Verification items for this drawing (mm, ordinates from the low corner). Round coordinates to 2 decimals unless told otherwise and drop trailing zeros. Order: outer loops, then holes, each group sorted by start corner. A loop starts at its lowest first (then second) coordinate and runs counter-clockwise, first axis right, second up. Notation, with made-up numbers: (65.25, 28.5) -> (87.25, 28.5) arc R20 ccw to (87.25, 45.5) -> close; hole circle Ø4 at (69, 89.25). An arc over 180 degrees is marked (long way). Put each result on its own line as item: value.
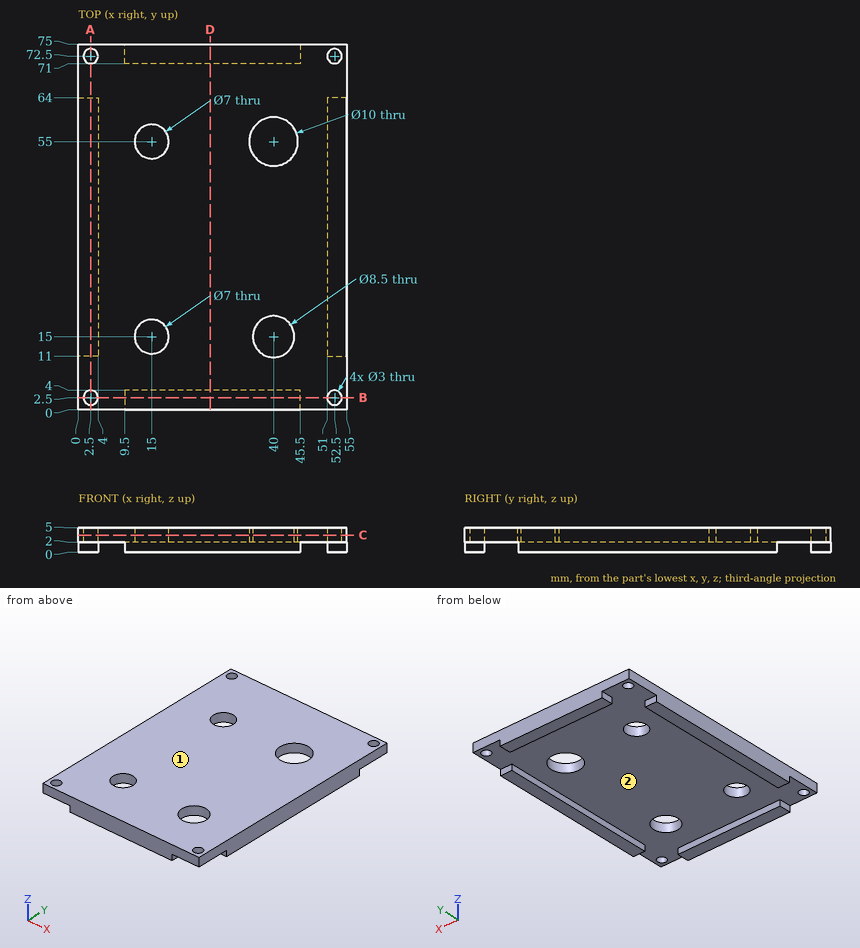
Item 1: Section check C-C on z = 3.5. State how many separate pieces and enclosed holes the cut face has, then the cut area to 3 significant figures.
Check sheet entries:
separate pieces: 1
enclosed holes: 8
area: 3,880 mm^2
Item 2: Section check D-D on x = 27. Record the boundary of the cut face in (y, z).
Check sheet entries:
outline: (0, 0) -> (4, 0) -> (4, 2) -> (71, 2) -> (71, 0) -> (75, 0) -> (75, 5) -> (0, 5) -> close
Item 3: Section check B-B on y = 2.5. Record the boundary of the cut face in (x, z).
Check sheet entries:
outline: (0, 2) -> (1, 2) -> (1, 5) -> (0, 5) -> close; (4, 2) -> (9.5, 2) -> (9.5, 0) -> (45.5, 0) -> (45.5, 2) -> (51, 2) -> (51, 5) -> (4, 5) -> close; (54, 2) -> (55, 2) -> (55, 5) -> (54, 5) -> close
Item 4: Material ranges on L1, parallel to Y at x = 2.5, z = 3.8; L2, parallel to Y at x = 40, z = 2.85; L3, parallel to X at y = 72.5, z = 4.15, recorded low to high. Write a range as [from, to].
Check sheet entries:
L1: y = [0, 1], [4, 71], [74, 75]
L2: y = [0, 10.75], [19.25, 50], [60, 75]
L3: x = [0, 1], [4, 51], [54, 55]
Item 5: Gauge pin test, flat ends, axial feed: pin 1 Ø1.6 at (y, z) = (72.5, 1) entering from +X; pin 2 Ø2 at (x, y) = (16, 34.5) entering from -Z; pin 3 Ø1 at (x, z) = (1.5, 0.5) entering from +Y; pin 4 Ø2.5 at (x, y) = (52.5, 72.5) entering from -Z. Record the tip position at first contact, or that the pin passes through.
Check sheet entries:
pin 1: stops at x = 45.5
pin 2: stops at z = 2
pin 3: stops at y = 64
pin 4: passes through
Item 6: Section check A-A on x = 2.5. Record the boundary of the cut face in (y, z).
Check sheet entries:
outline: (0, 2) -> (1, 2) -> (1, 5) -> (0, 5) -> close; (4, 2) -> (11, 2) -> (11, 0) -> (64, 0) -> (64, 2) -> (71, 2) -> (71, 5) -> (4, 5) -> close; (74, 2) -> (75, 2) -> (75, 5) -> (74, 5) -> close
Item 7: Release check for a two-part mould opening along Y. For the marked faces 1 and 2 record: +Y half, -Y half, draft (parallel to the pull), parting line (faces both ways), or undercut.
Check sheet entries:
face 1: draft
face 2: undercut
